Work out the finished part from the listing and answer in its coordinate system (mm). A direction names the side the tool comes from. Round coordinates to 2 decimals unless told otherwise and drop trailing zeros. Write each loop counter-clockwise with the first axis right and the second up, starting at its lowest first coordinate (ties: lowest second). Pieces come first, ordered by that corner, then holes. Notation, with made-up numbers: M 70,-20 L 127,-20 A17 cw 127,-1 Z; hole C 67.25,29 d7. An arc over 180 degrees is marked long. Answer in a Markdown table with one row per item.
```python
from build123d import *

# Parameters (mm, degrees)
SALIENTE_EXTRUIR1_DEPTH = 3
CROQUIS2_R              = 2.5
SALIENTE_EXTRUIR2_DEPTH = 10
CROQUIS3_R              = 1.5
SALIENTE_EXTRUIR3_DEPTH = 10


with BuildPart() as part:
    # Croquis1 → Saliente-Extruir1 (new body)
    with BuildSketch(Plane(origin=(0, 0, 0), x_dir=(1, 0, 0), z_dir=(0, 1, 0))):
        with BuildLine():
            Line((-15.839745962, 0), (15.839745962, 0))
            ThreePointArc((15.839745962, 0), (20.169872981, 2.5), (20.169872981, 7.5))
            Line((20.169872981, 7.5), (4.330127019, 34.935244785))
            ThreePointArc((4.330127019, 34.935244785), (0, 37.435244785), (-4.330127019, 34.935244785))
            Line((-4.330127019, 34.935244785), (-20.169872981, 7.5))
            ThreePointArc((-20.169872981, 7.5), (-20.169872981, 2.5), (-15.839745962, 0))
        make_face()
    extrude(amount=SALIENTE_EXTRUIR1_DEPTH)

    # Croquis2 → Saliente-Extruir2 (add)
    with BuildSketch(Plane(origin=(0, 3, 0), x_dir=(1, 0, 0), z_dir=(0, 1, 0))):
        with Locations(Location((0, 32.435244785, 0), (0, 0, 270))):
            Circle(CROQUIS2_R)
        with Locations(Location((15.839745962, 5, 0), (0, 0, 270))):
            Circle(CROQUIS2_R)
        with Locations(Location((-15.839745962, 5, 0), (0, 0, 270))):
            Circle(CROQUIS2_R)
    extrude(amount=SALIENTE_EXTRUIR2_DEPTH)

    # Croquis3 → Saliente-Extruir3 (add)
    with BuildSketch(Plane(origin=(0, 3, 0), x_dir=(1, 0, 0), z_dir=(0, 1, 0))):
        with Locations(Location((0.008103959, 13.990369441, 0), (0, 0, 270))):
            Circle(CROQUIS3_R)
    extrude(amount=SALIENTE_EXTRUIR3_DEPTH)


solid = part.part
```
1. The part is cut by section A-A (z = -5). Determine the outline of the cut face in (x, y).
Calculated:
| item | result |
|---|---|
| outline | M -20.84,0 L 20.84,0 L 20.84,3 L 18.34,3 L 18.34,13 L 13.34,13 L 13.34,3 L -13.34,3 L -13.34,13 L -18.34,13 L -18.34,3 L -20.84,3 Z |
2. Given pin 1 (6 mm diameter, centred on x = -0.5, z = -13.5, fed in from -Y); pin 2 (5 mm diameter, centred on x = 12, y = 7, fed in from +Z); pin 3 (1.5 mm diameter, centred on y = 5.5, z = -18, fed in from -X), each flat-ended and moving along its own axis, determine where each tip first touches the part or whether it passes through.
Calculated:
| item | result |
|---|---|
| pin 1 | stops at y = 0 |
| pin 2 | stops at z = -2.89 |
| pin 3 | passes through |
3. The part is cut by section D-D (z = -14.5). Determine the outline of the cut face in (x, y), plus the area to 3 significant figures.
Calculated:
| item | result |
|---|---|
| outline | M -16.13,0 L 16.13,0 L 16.13,3 L 1.42,3 L 1.42,13 L -1.4,13 L -1.4,3 L -16.13,3 Z |
| area | 125 mm² |
4. Consider line 1 along Y through (x, z) = (3.5, -30); line 2 along X through (y, z) = (9.5, -7); line 3 along X through (y, z) = (4.75, -13). Determine where each line is inside the solid, lowest interval first. Write a range as from..to.
Calculated:
| item | result |
|---|---|
| line 1 | y = 0..3 |
| line 2 | x = -17.34..-14.34, 14.34..17.34 |
| line 3 | x = -1.12..1.13 |
5. A tool of negligible diameter and unlimited length cuts with its end or side. For faces 1 (the flat face through (-12.14, 1.48, -21.41)), 2 (the flat face through (0, 3, -11)), from which of +Z, -Z, +X, -X, +Y, -Y can it reach the whole face along a straight path? Write none if from no direction.
Calculated:
| item | result |
|---|---|
| face 1 | -Z, -X, +Y, -Y |
| face 2 | +Y |
6. The part is cut by section C-C (y = 5.5). Determine the outline of the cut face in (x, z), plus the area to 3 significant figures.
Calculated:
| item | result |
|---|---|
| outline | C -15.84,-5 d5; C 0,-32.44 d5; C 0.01,-13.99 d3; C 15.84,-5 d5 |
| area | 66.0 mm² |
7. The part is cut by section B-B (x = -17). Determine the outline of the cut face in (y, z).
Calculated:
| item | result |
|---|---|
| outline | M 0,-12.99 L 3,-12.99 L 3,-7.21 L 13,-7.21 L 13,-2.79 L 3,-2.79 L 3,-0.14 L 0,-0.14 Z |
8. Determine the mould class of faces 3 (the cylindrical face through (0.07, 7.93, -15.49)), 4 (the flat face through (0, 0, -15)), 5 (the cylindrical face through (20.133, 1.479, -2.437)) for opening direction Z: released by +Z, released by -Z, zero draft, split by the parting line, or undercut.
Calculated:
| item | result |
|---|---|
| face 3 | undercut |
| face 4 | zero draft |
| face 5 | split by the parting line |
